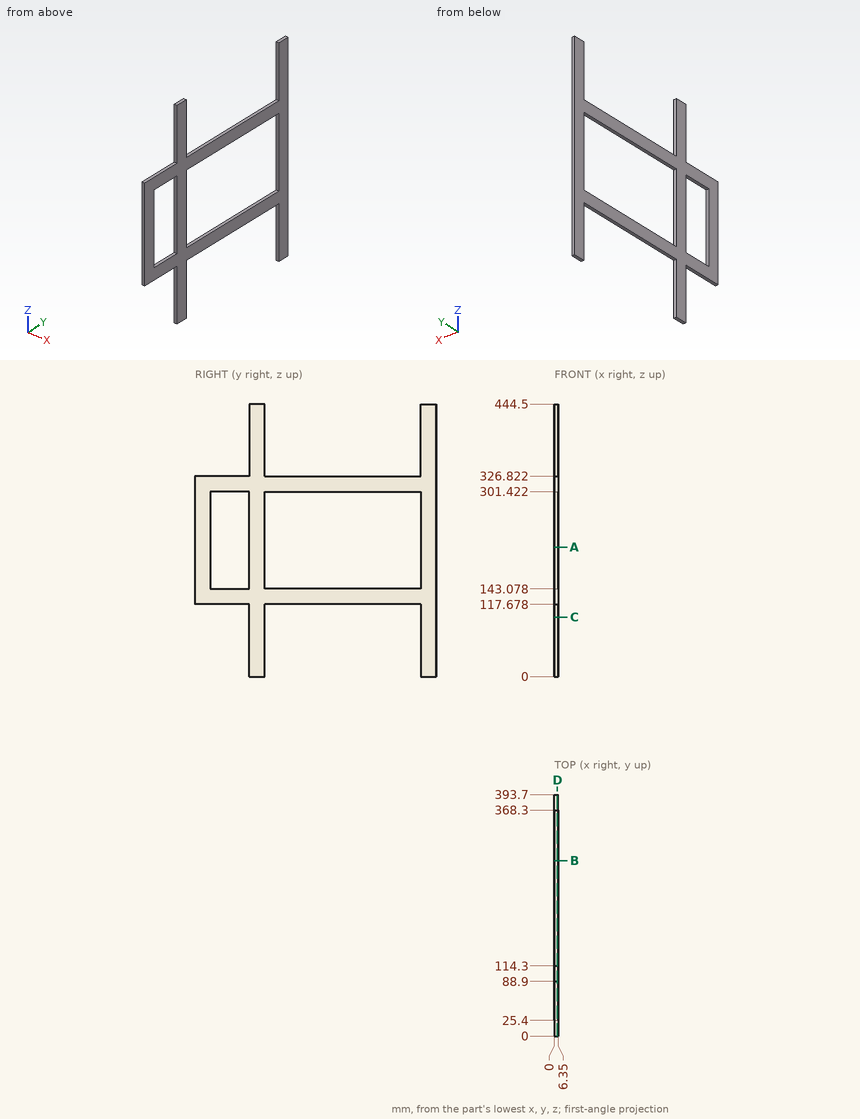
Check sheet for the drawn part. Datum: minimum x, y, z corner. Units: mm. Round coordinates to 2 decimals unless told otherwise and drop trailing zeros. Order: outer loops, then holes, each group sorted by start corner. A loop starts at its lowest first (then second) coordinate and runs counter-clockwise, first axis right, second up.
(1) Scan lines: probe 1 along Y at (x, z) = (1.5, 226.5); probe 2 along Y at (x, z) = (2.5, 105.5); probe 3 along Z at (x, y) = (3, 254.5). Record each from-to range of solid material in increasing order.
(2) Cross-section at C-C, the plane z = 97. Enter the section's corners in (x, y), and give its area (3 significant figures).
(3) Go/stop test with flat-tipped pins: P1, Ø1.9, axis at x = 3, y = 230, coming from the +Z side; P2, Ø1, axis at x = 3.5, z = 90, coming from the -Y side. Record where each tip stops, or that it passes through.
(4) Cross-section at D-D, the plane x = 5.25. Enter the section's corners in (y, z).
(5) Cross-section at B-B, the plane y = 286. Enter the section's corners in (x, z).
(6) Cross-section at A-A, the plane z = 211. Enter the section's corners in (x, y).
Check sheet entries:
1. probe 1: y = 0 to 25.4, 88.9 to 114.3, 368.3 to 393.7
1. probe 2: y = 88.9 to 114.3, 368.3 to 393.7
1. probe 3: z = 117.68 to 143.08, 301.42 to 326.82
2. outline: (0, 88.9) - (6.35, 88.9) - (6.35, 114.3) - (0, 114.3) - close; (0, 368.3) - (6.35, 368.3) - (6.35, 393.7) - (0, 393.7) - close
2. area: 323 mm2
3. P1: stops at z = 326.82
3. P2: stops at y = 88.9
4. outline: (0, 117.68) - (88.9, 117.68) - (88.9, 0) - (114.3, 0) - (114.3, 117.68) - (368.3, 117.68) - (368.3, 0) - (393.7, 0) - (393.7, 444.5) - (368.3, 444.5) - (368.3, 326.82) - (114.3, 326.82) - (114.3, 444.5) - (88.9, 444.5) - (88.9, 326.82) - (0, 326.82) - close; hole (25.4, 143.08) - (88.9, 143.08) - (88.9, 301.42) - (25.4, 301.42) - close; hole (114.3, 143.08) - (368.3, 143.08) - (368.3, 301.42) - (114.3, 301.42) - close
5. outline: (0, 117.68) - (6.35, 117.68) - (6.35, 143.08) - (0, 143.08) - close; (0, 301.42) - (6.35, 301.42) - (6.35, 326.82) - (0, 326.82) - close
6. outline: (0, 0) - (6.35, 0) - (6.35, 25.4) - (0, 25.4) - close; (0, 88.9) - (6.35, 88.9) - (6.35, 114.3) - (0, 114.3) - close; (0, 368.3) - (6.35, 368.3) - (6.35, 393.7) - (0, 393.7) - close
